Source: CAD feature listing. Evaluate the final solid. Frame: model axes, mm. Round coordinates to 2 decimals unless told otherwise and drop trailing zeros. Order: outer loops, then holes, each group sorted by start corner. A loop starts at its lowest first (then second) coordinate and runs counter-clockwise, first axis right, second up. Notation, with made-up numbers: (86.25, -39) - (141.25, -39) arc R32 ccw to (141.25, 0) - close; hole circle Ø6 at (-30.75, -13). An arc over 180 degrees is marked (long way). Return JSON: item names as keys, results as strings. Group by question number.
1) Ray query, line 1 (Z direction, x = 45.5, y = -12); line 2 (X direction, y = 30.5, z = 36.5); line 3 (X direction, y = -30.5, z = 142). Return the intervals inside material, ascending. Write a range as from..to.
2) Section A-A, the plane y = -14. Return loops of the section in (x, z), plus the area to 3 significant figures.
3) Section B-B, the plane x = -59. Give the number of separate pieces and of enclosed holes in the cut face, plus the area to 3 significant figures.
4) Contact query for flat-ended pins moving along their axis: P1, Ø6, axis at y = -22, z = 141, coming from the +X side; P2, Ø4, axis at x = -26, y = -5, coming from the +Z side; P3, Ø2, axis at y = -31.5, z = 140, coming from the +X side. Output: stop coordinate, or through.
```python
from build123d import *

# Parameters (mm, degrees)
SKETCH_1_W      = 230
SKETCH_1_H      = 110
SKETCH_1_R      = 3
REVOLVE_1_ANGLE = 90


with BuildPart() as part:
    # 草图1 → 旋转1 (revolve)
    with BuildSketch(Plane.XY):
        Rectangle(SKETCH_1_W, SKETCH_1_H)
        with Locations((-105, 45)):
            Circle(SKETCH_1_R, mode=Mode.SUBTRACT)
        with Locations((-105, -45)):
            Circle(SKETCH_1_R, mode=Mode.SUBTRACT)
        with Locations((105, -45)):
            Circle(SKETCH_1_R, mode=Mode.SUBTRACT)
        with Locations((105, 45)):
            Circle(SKETCH_1_R, mode=Mode.SUBTRACT)
    revolve(axis=Axis((-115, 55, 0), (0, -1, 0)), revolution_arc=REVOLVE_1_ANGLE)


solid = part.part
```
Geometry check:
{
 "1": {"line 1": "0..164.74", "line 2": "-115..112.09", "line 3": "-115..65.93"},
 "2": {"outline": "(-115, 0) - (115, 0) arc R230 ccw to (-115, 230) - close", "area": "41,500 mm2"},
 "3": {"separate pieces": "1", "enclosed holes": "2", "area": "24,500 mm2"},
 "4": {"P1": "x = 69", "P2": "z = 212.91", "P3": "x = 68.25"}
}
